Part model, mm, in its own coordinate system. Face numbers are marked on the shaded views. A direction names the side the tool comes from. Coordinates: 2 decimals unless noted, no trailing zeros. Write each loop counter-clockwise with the first axis right and the second up, starting at its lowest first coordinate (ties: lowest second). Pieces come first, ordered by that corner, then holes. Notation, with made-up numbers: (-3, 48.25) -> (7, 48.25) arc R9 cw to (7, 55.25) -> close; hole circle Ø5 at (79, 44). An arc over 180 degrees is marked (long way). One line per question, with ' | ' between items. Start each with the question number.
Item 1: 3-axis set-ups, long thin cutter, end or side, ignore diameter. For the marked faces 1 and 2: which of +Z, -Z, +X, -X, +Y, -Y reach the whole face in a straight line?
Item 2: Saw through at A-A (z = 16). List the corners of the cut face in (x, y).
Item 3: Saw through at B-B (x = 9). List the corners of the cut face in (y, z).
Item 4: Pin check, flat tips, straight feed: pin 1 (5 mm diameter, centred on y = 16.5, z = 15.5, fed in from -X); pin 2 (1 mm diameter, centred on x = 4, z = 12, fed in from +Y). Stop position of each tip, or through.
Item 5: Saw through at C-C (z = 18.75). List the corners of the cut face in (x, y).
Item 6: Probe probe 1 along Z at (x, y) = (18.45, 50); probe 2 along Z at (x, y) = (10, 2.35); probe 3 along X at (y, z) = (1.1, 16). List the from-to ranges inside material, lowest first. Write a range as [from, to].
Item 7: Saw through at D-D (y = 47). List the corners of the cut face in (x, z), and give its area (3 significant figures).
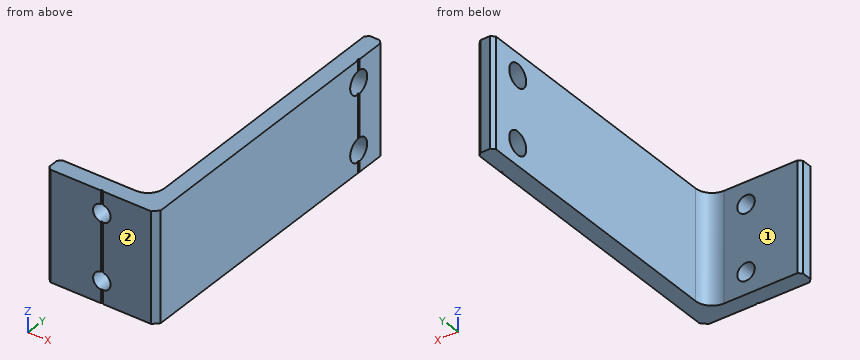
from build123d import *

# Parameters (mm, degrees)
EXTRUDE_1_DEPTH     = 20
FILLET_1_R          = 3
SKETCH_2_R          = 2.1
CUT_EXTRUDE_1_DEPTH = 20
SKETCH_3_R          = 1.6
CUT_EXTRUDE_2_DEPTH = 20
CHAMFER_1_SIZE      = 1
CHAMFER_2_SIZE      = 0.6
SKETCH_4_R          = 0.2
CUT_EXTRUDE_3_DEPTH = 32


with BuildPart() as part:
    # 草图1 → 凸台-拉伸1 (new body)
    with BuildSketch(Plane.XY):
        Polygon((0, 0), (20, 0), (20, 56), (17, 56), (17, 3), (0, 3), align=None)
    extrude(amount=EXTRUDE_1_DEPTH)

    # 圆角1
    fillet_1_edges = [part.edges().sort_by_distance(p)[0] for p in [
        (17, 3, 10),
    ]]
    fillet(fillet_1_edges, radius=FILLET_1_R)

    # 草图2 → 切除-拉伸1 (cut)
    with BuildSketch(Plane.ZY.offset(-17)):
        with Locations((4, 50)):
            Circle(SKETCH_2_R)
        with Locations((16, 50)):
            Circle(SKETCH_2_R)
    extrude(amount=-CUT_EXTRUDE_1_DEPTH, mode=Mode.SUBTRACT)

    # 草图3 → 切除-拉伸2 (cut)
    with BuildSketch(Plane(origin=(0, 3, 0), x_dir=(1, 0, 0), z_dir=(0, 1, 0))):
        with Locations((10, -4)):
            Circle(SKETCH_3_R)
        with Locations((10, -16)):
            Circle(SKETCH_3_R)
    extrude(amount=-CUT_EXTRUDE_2_DEPTH, mode=Mode.SUBTRACT)

    # 倒角1
    chamfer_1_edges = [part.edges().sort_by_distance(p)[0] for p in [
        (20, 0, 10),
    ]]
    chamfer(chamfer_1_edges, length=CHAMFER_1_SIZE)

    # 倒角2
    chamfer_2_edges = [part.edges().sort_by_distance(p)[0] for p in [
        (0, 3, 10),
        (17, 56, 10),
        (20, 56, 10),
        (0, 0, 10),
    ]]
    chamfer(chamfer_2_edges, length=CHAMFER_2_SIZE)

    # 草图4 → 切除-拉伸3 (cut)
    with BuildSketch(Plane.XY.offset(20)):
        with Locations((10, 0)):
            Circle(SKETCH_4_R)
        with Locations((20, 50)):
            Circle(SKETCH_4_R)
    extrude(amount=-CUT_EXTRUDE_3_DEPTH, mode=Mode.SUBTRACT)


solid = part.part
From the geometry:
1) face 1: +Z, -Z, -X, +Y | face 2: +Z, -Z, +X, -X, -Y
2) outline: (0, 0.6) -> (0.6, 0) -> (8.4, 0) -> (8.4, 3) -> (0.6, 3) -> (0, 2.4) -> close; (11.6, 0) -> (19, 0) -> (20, 1) -> (20, 47.9) -> (17, 47.9) -> (17, 6) arc R3 cw to (14, 3) -> (11.6, 3) -> close; (17, 52.1) -> (20, 52.1) -> (20, 55.4) -> (19.4, 56) -> (17.6, 56) -> (17, 55.4) -> close
3) outline: (0, 0) -> (3, 0) -> (3, 2.75) -> (0, 2.75) -> close; (0, 5.25) -> (3, 5.25) -> (3, 14.75) -> (0, 14.75) -> close; (0, 17.25) -> (3, 17.25) -> (3, 20) -> (0, 20) -> close
4) pin 1: x = 17 | pin 2: y = 3
5) outline: (0, 0.6) -> (0.6, 0) -> (9.8, 0) arc R0.2 cw to (10.2, 0) -> (19, 0) -> (20, 1) -> (20, 49.8) arc R0.2 cw to (20, 50.2) -> (20, 55.4) -> (19.4, 56) -> (17.6, 56) -> (17, 55.4) -> (17, 6) arc R3 cw to (14, 3) -> (0.6, 3) -> (0, 2.4) -> close
6) probe 1: [0, 1.9], [6.1, 13.9], [18.1, 20] | probe 2: [0, 2.4], [5.6, 14.4], [17.6, 20] | probe 3: [0, 8.4], [11.6, 20]
7) outline: (17, 0) -> (20, 0) -> (20, 20) -> (17, 20) -> close | area: 60.0 mm2
